from build123d import *

# Parameters (mm, degrees)
CROQUIS1_W              = 100
CROQUIS1_H              = 49
SALIENTE_EXTRUIR1_DEPTH = 40
CROQUIS2_W              = 70
CROQUIS2_H              = 29
CORTAR_EXTRUIR1_DEPTH   = 35
CORTAR_EXTRUIR2_DEPTH   = 14.9
CORTAR_EXTRUIR4_DEPTH   = 119.325821358
CROQUIS6_W              = 20.5
CROQUIS6_H              = 16.2
CORTAR_EXTRUIR6_DEPTH   = 119.325821358
CROQUIS7_W              = 58
CROQUIS7_H              = 18
SALIENTE_EXTRUIR2_DEPTH = 16
CROQUIS8_W              = 54
CROQUIS8_H              = 14
CORTAR_EXTRUIR7_DEPTH   = 16
ENVOLVER2_START         = -2.5
ENVOLVER2_DEPTH         = 2.5
CROQUIS11_W             = 75
CROQUIS11_H             = 10
SALIENTE_EXTRUIR3_DEPTH = 44
CROQUIS12_W             = 67
CROQUIS12_H             = 45
CORTAR_EXTRUIR8_DEPTH   = 5
CROQUIS13_W             = 71
CROQUIS13_H             = 1.5
CORTAR_EXTRUIR9_DEPTH   = 54
CROQUIS14_W             = 20
CROQUIS14_H             = 12
CORTAR_EXTRUIR10_DEPTH  = 5
CORTAR_EXTRUIR11_REACH  = 144.299
CROQUIS5_W              = 20.5
CROQUIS5_H              = 16.2
CROQUIS15_W             = 75
CROQUIS15_H             = 10
SALIENTE_EXTRUIR4_DEPTH = 1
CROQUIS16_W             = 75
CROQUIS16_H             = 14.9
CROQUIS16_W_2           = 15
CROQUIS16_H_2           = 25
CORTAR_EXTRUIR12_DEPTH  = 2.4
SALIENTE_EXTRUIR5_DEPTH = 2


# Read off the part's stored shape, not the designer's step: Envolver2
with BuildPart() as part:
    # Croquis1 → Saliente-Extruir1 (new body)
    with BuildSketch(Plane(origin=(0, 0, 0), x_dir=(1, 0, 0), z_dir=(0, 1, 0))):
        with Locations((50, 24.5)):
            Rectangle(CROQUIS1_W, CROQUIS1_H)
    extrude(amount=SALIENTE_EXTRUIR1_DEPTH)

    # Croquis2 → Cortar-Extruir1 (cut)
    with BuildSketch(Plane(origin=(0, 40, 0), x_dir=(1, 0, 0), z_dir=(0, 1, 0))):
        with Locations((50, 29.5)):
            Rectangle(CROQUIS2_W, CROQUIS2_H)
    extrude(amount=-CORTAR_EXTRUIR1_DEPTH, mode=Mode.SUBTRACT)

    # Croquis3 → Cortar-Extruir2 (cut)
    with BuildSketch(Plane.XY):
        Polygon((12.5, 5), (12.5, 25), (87.5, 25), (87.5, 5), (100, 5), (100, 40), (0, 40), (0, 5), align=None)
    extrude(amount=-CORTAR_EXTRUIR2_DEPTH, mode=Mode.SUBTRACT)

    # Croquis4 → Cortar-Extruir4 (cut, through all)
    with BuildSketch(Plane.ZY):
        Polygon((-44, 25), (-19, 25), (-19, 5), (-14.9, 5), (-14.9, 40), (-44, 40), align=None)
    extrude(amount=-CORTAR_EXTRUIR4_DEPTH, mode=Mode.SUBTRACT)

    # Croquis6 → Cortar-Extruir6 (cut, through all)
    with BuildSketch(Plane(origin=(100, 0, 0), x_dir=(0, 0, -1), z_dir=(1, 0, 0))):
        with Locations((31.75, 14.5)):
            Rectangle(CROQUIS6_W, CROQUIS6_H)
    extrude(amount=-CORTAR_EXTRUIR6_DEPTH, mode=Mode.SUBTRACT)

    # Croquis7 → Saliente-Extruir2 (add)
    with BuildSketch(Plane(origin=(0, 5, 0), x_dir=(1, 0, 0), z_dir=(0, 1, 0))):
        with Locations((50, 35)):
            Rectangle(CROQUIS7_W, CROQUIS7_H)
    extrude(amount=SALIENTE_EXTRUIR2_DEPTH)

    # Croquis8 → Cortar-Extruir7 (cut)
    with BuildSketch(Plane(origin=(0, 21, 0), x_dir=(1, 0, 0), z_dir=(0, 1, 0))):
        with Locations((50, 35)):
            Rectangle(CROQUIS8_W, CROQUIS8_H)
    extrude(amount=-CORTAR_EXTRUIR7_DEPTH, mode=Mode.SUBTRACT)

    # Envolver2 outline → Envolver2 (cut)
    # profile 1 of 3: a face of its own
    with BuildSketch(Plane(origin=(0, 5, 0), x_dir=(1, 0, 0), z_dir=(0, 1, 0)).offset(ENVOLVER2_START)):
        with BuildLine():
            add(Edge.make_bspline(
                [(44.845927513, 22.682039813), (44.880502524, 22.681581101), (44.94779002, 22.680688388), (45.045978034, 22.678103561), (45.138406194, 22.671034857), (45.225422346, 22.663758255), (45.306894242, 22.652117669), (45.382891805, 22.638865253), (45.453428219, 22.622573117), (45.519399834, 22.604194379), (45.582065701, 22.58175166), (45.642294727, 22.553081251), (45.700763218, 22.518735345), (45.757273689, 22.477750733), (45.813128977, 22.432374893), (45.865885411, 22.37921084), (45.918377238, 22.321807714), (45.967578278, 22.25830401), (46.01447324, 22.191680732), (46.054376208, 22.120908747), (46.088223994, 22.047966819), (46.117214563, 21.973058038), (46.136979973, 21.894799291), (46.154181469, 21.814812457), (46.162464556, 21.732060085), (46.163897144, 21.676148523), (46.164618555, 21.647993057)],
                knots=[0, 0, 0, 0, 0.054369818, 0.105810783, 0.1543913, 0.200099433, 0.243069893, 0.283740822, 0.321360744, 0.356845277, 0.391373506, 0.42587086, 0.461574928, 0.497826917, 0.535543491, 0.574581255, 0.615459073, 0.657779879, 0.700797841, 0.743450957, 0.785305491, 0.827181235, 0.869502041, 0.912065543, 0.955718718, 1, 1, 1, 1], degree=3))
            Line((44.845927513, 22.682039813), (43.424314244, 22.682039813))
            Line((43.424314244, 22.682039813), (42.805172718, 18.976839617))
            Line((42.805172718, 18.976839617), (43.469342719, 18.976839617))
            Line((43.469342719, 18.976839617), (43.718607489, 20.469211918))
            Line((43.718607489, 20.469211918), (44.603095383, 20.469211918))
            Line((44.603095383, 20.469211918), (45.04292709, 18.976839617))
            Line((45.04292709, 18.976839617), (45.752929645, 18.976839617))
            Line((45.752929645, 18.976839617), (45.28977962, 20.548011749))
            add(Edge.make_bspline(
                [(46.164618555, 21.647993057), (46.164091676, 21.617670303), (46.163039403, 21.5571103), (46.151744736, 21.467468845), (46.13622668, 21.379126232), (46.112503265, 21.292592771), (46.082048693, 21.207680933), (46.044780457, 21.124441143), (46.001130757, 21.043108672), (45.951712013, 20.9635574), (45.895224481, 20.887990565), (45.830214645, 20.819272615), (45.758276279, 20.757071565), (45.678885267, 20.701205138), (45.592072867, 20.652370985), (45.497799172, 20.610367641), (45.396617343, 20.574987864), (45.325850603, 20.557119534), (45.28977962, 20.548011749)],
                knots=[0, 0, 0, 0, 0.059520551, 0.118873267, 0.177208837, 0.235565778, 0.294841411, 0.354222133, 0.414510544, 0.476000381, 0.538010758, 0.599455515, 0.661405537, 0.724496825, 0.78978963, 0.856706752, 0.926961053, 1, 1, 1, 1], degree=3))
        make_face()
        with BuildLine():
            add(Edge.make_bspline(
                [(44.743809366, 21.03528417), (44.778129381, 21.03600119), (44.843652036, 21.0373701), (44.937526666, 21.044910102), (45.022020151, 21.059216882), (45.097465695, 21.079213334), (45.164300411, 21.104537257), (45.221481868, 21.136836672), (45.270624581, 21.17399479), (45.32077283, 21.232312946), (45.36864261, 21.310567266), (45.413007527, 21.407196099), (45.438530205, 21.507321555), (45.442292151, 21.574957755), (45.444162962, 21.608593141)],
                knots=[0, 0, 0, 0, 0.099664188, 0.190275618, 0.273183536, 0.348129931, 0.416633313, 0.480054439, 0.538277477, 0.594505454, 0.702244126, 0.80362549, 0.902343236, 1, 1, 1, 1], degree=3))
            Line((44.743809366, 21.03528417), (43.812684837, 21.03528417))
            Line((43.812684837, 21.03528417), (43.993602816, 22.115967561))
            Line((43.993602816, 22.115967561), (44.735768567, 22.115967561))
            add(Edge.make_bspline(
                [(45.444162962, 21.608593141), (45.443321191, 21.636863214), (45.441681994, 21.691914124), (45.421908744, 21.770970842), (45.392768442, 21.844328967), (45.35019923, 21.909220717), (45.300609579, 21.965653441), (45.246923641, 22.013950522), (45.187891151, 22.050903022), (45.122329195, 22.077622199), (45.046506806, 22.09459194), (44.957252302, 22.107151834), (44.85196106, 22.115045121), (44.776255138, 22.115646142), (44.735768567, 22.115967561)],
                knots=[0, 0, 0, 0, 0.084973229, 0.165470167, 0.24404472, 0.32176826, 0.397881214, 0.469968558, 0.538528016, 0.606605512, 0.682202732, 0.771959831, 0.878046995, 1, 1, 1, 1], degree=3))
        make_face(mode=Mode.SUBTRACT)
    # profile 2 of 3: a face of its own
    with BuildSketch(Plane(origin=(0, 5, 0), x_dir=(1, 0, 0), z_dir=(0, 1, 0)).offset(ENVOLVER2_START)):
        Polygon((46.976739258, 22.682039813), (46.357597732, 18.976839617), (48.79395984, 18.976839617), (48.892057588, 19.542911869), (47.113432841, 19.542911869), (47.285505941, 20.572134146), (48.696666171, 20.572134146), (48.78913536, 21.138206398), (47.379583289, 21.138206398), (47.54281151, 22.115967561), (49.257109864, 22.115967561), (49.355207612, 22.682039813), align=None)
    # profile 3 of 3: a face of its own
    with BuildSketch(Plane(origin=(0, 5, 0), x_dir=(1, 0, 0), z_dir=(0, 1, 0)).offset(ENVOLVER2_START)):
        Polygon((50.984273497, 22.682039813), (49.96148386, 22.682039813), (49.342342334, 18.976839617), (49.858561632, 18.976839617), (50.417397165, 22.321007936), (50.952914381, 18.976839617), (51.313946257, 18.976839617), (52.891551028, 22.350758892), (52.327086936, 18.976839617), (52.991256936, 18.976839617), (53.611202541, 22.682039813), (52.559466028, 22.682039813), (51.387921608, 20.172506434), align=None)
    extrude(amount=ENVOLVER2_DEPTH, mode=Mode.SUBTRACT)

    # Croquis11 → Saliente-Extruir3 (add)
    with BuildSketch(Plane(origin=(0, 0, -49), x_dir=(-1, 0, 0), z_dir=(0, 0, -1))):
        with Locations((-50, 35)):
            Rectangle(CROQUIS11_W, CROQUIS11_H)
    extrude(amount=SALIENTE_EXTRUIR3_DEPTH)

    # Croquis12 → Cortar-Extruir8 (cut)
    with BuildSketch(Plane(origin=(0, 40, 0), x_dir=(1, 0, 0), z_dir=(0, 1, 0))):
        with Locations((50, 66.5)):
            Rectangle(CROQUIS12_W, CROQUIS12_H)
    extrude(amount=-CORTAR_EXTRUIR8_DEPTH, mode=Mode.SUBTRACT)

    # Croquis13 → Cortar-Extruir9 (cut)
    with BuildSketch(Plane.XY.offset(-44)):
        with Locations((50, 37.5)):
            Rectangle(CROQUIS13_W, CROQUIS13_H)
    extrude(amount=-CORTAR_EXTRUIR9_DEPTH, mode=Mode.SUBTRACT)

    # Croquis14 → Cortar-Extruir10 (cut)
    with BuildSketch(Plane(origin=(0, 35, 0), x_dir=(1, 0, 0), z_dir=(0, 1, 0))):
        with Locations((50.5, 80)):
            Rectangle(CROQUIS14_W, CROQUIS14_H)
    extrude(amount=-CORTAR_EXTRUIR10_DEPTH, mode=Mode.SUBTRACT)

    # Croquis5 → Cortar-Extruir11 (cut, up to next)
    with BuildSketch(Plane.XY, mode=Mode.PRIVATE) as cortar_extruir11_sk1:
        with Locations((26.25, 14.5)):
            Rectangle(CROQUIS5_W, CROQUIS5_H)
    cortar_extruir11_tool1 = extrude(cortar_extruir11_sk1.sketch, amount=-CORTAR_EXTRUIR11_REACH, mode=Mode.PRIVATE) & part.part
    # Croquis5 → Cortar-Extruir11 (cut, up to next)
    with BuildSketch(Plane.XY, mode=Mode.PRIVATE) as cortar_extruir11_sk2:
        with Locations((50, 14.5)):
            Rectangle(CROQUIS5_W, CROQUIS5_H)
    cortar_extruir11_tool2 = extrude(cortar_extruir11_sk2.sketch, amount=-CORTAR_EXTRUIR11_REACH, mode=Mode.PRIVATE) & part.part
    # Croquis5 → Cortar-Extruir11 (cut, up to next)
    with BuildSketch(Plane.XY, mode=Mode.PRIVATE) as cortar_extruir11_sk3:
        with Locations((73.75, 14.5)):
            Rectangle(CROQUIS5_W, CROQUIS5_H)
    cortar_extruir11_tool3 = extrude(cortar_extruir11_sk3.sketch, amount=-CORTAR_EXTRUIR11_REACH, mode=Mode.PRIVATE) & part.part
    add(cortar_extruir11_tool1.solids().sort_by_distance((26.25, 14.5, 0))[0], mode=Mode.SUBTRACT)
    add(cortar_extruir11_tool2.solids().sort_by_distance((50, 14.5, 0))[0], mode=Mode.SUBTRACT)
    add(cortar_extruir11_tool3.solids().sort_by_distance((73.75, 14.5, 0))[0], mode=Mode.SUBTRACT)

    # Croquis15 → Saliente-Extruir4 (add)
    with BuildSketch(Plane(origin=(0, 0, -93), x_dir=(-1, 0, 0), z_dir=(0, 0, -1))):
        with Locations((-50, 35)):
            Rectangle(CROQUIS15_W, CROQUIS15_H)
    extrude(amount=SALIENTE_EXTRUIR4_DEPTH)

    # Croquis16 → Cortar-Extruir12 (cut)
    with BuildSketch(Plane(origin=(0, 25, 0), x_dir=(1, 0, 0), z_dir=(0, 1, 0))):
        with Locations((50, 7.45)):
            Rectangle(CROQUIS16_W, CROQUIS16_H)
        with Locations((7.5, 31.5)):
            Rectangle(CROQUIS16_W_2, CROQUIS16_H_2)
        with Locations((92.5, 31.5)):
            Rectangle(CROQUIS16_W_2, CROQUIS16_H_2)
    extrude(amount=-CORTAR_EXTRUIR12_DEPTH, mode=Mode.SUBTRACT)

    # Croquis17 → Saliente-Extruir5 (add)
    with BuildSketch(Plane.XY.offset(-44)):
        Polygon((0, 40), (16.5, 40), (16.5, 38.25), (14.5, 38.25), (14.5, 36.75), (16.5, 36.75), (16.5, 35), (83.5, 35), (83.5, 36.75), (85.5, 36.75), (85.5, 38.25), (83.5, 38.25), (83.5, 40), (100, 40), (100, 22.6), (85, 22.6), (85, 5), (79, 5), (79, 21), (21, 21), (21, 5), (15, 5), (15, 22.6), (0, 22.6), align=None)
    extrude(amount=SALIENTE_EXTRUIR5_DEPTH)


solid = part.part
Verification items for the finished model (mm, model axes). A direction names the side the tool comes from. Give positions to 0.01 mm unless a question says otherwise; leave off trailing zeros. Loops run counter-clockwise (first coordinate to the right, second up) from the corner with the lowest first, then second, coordinate; pieces in that order, holes last.
1) Sectioned sample at B-B, the plane x = 70.5. Enter the section's corners in (y, z).
2) Sectioned sample at D-D, the plane z = -62. Enter the section's corners in (x, y).
3) Thickness scan on line 1 along Z through (x, y) = (14.5, 19.5); line 2 along Z through (x, y) = (48.5, 3.5); line 3 along X through (y, z) = (18, -39). Record the ranges inside material, lowest first.
4) Depth check by flat-ended pin: pin 1 Ø3 at (x, z) = (14, -7) entering from +Y; pin 2 Ø4.5 at (y, z) = (11.5, -11) entering from -X; pin 3 Ø7.5 at (x, z) = (48.5, -8) entering from +Y. Enter the tip coordinate at first touch or a pass-through.
5) Set-up check for faces 3 (the flat face through (93, 6.4, -32)), 4 (the flat face through (53, 6, -14.9)), 5 (the flat face through (92, 22.6, -20)), 6 (the flat face through (51, 30, -71)): record each of +Z, -Z, +X, -X, +Y, -Y from which the full face is reachable in a straight line by a thin tool's end or side.
6) Sectioned sample at A-A, the plane z = -38.5. Enter the section's corners in (x, y).
7) Sectioned sample at C-C, the plane y = 17. Count the separate pieces of the cut face and the enclosed holes in it, then the cut area to 3 significant figures.
8) Draft check along Z on faces 1 (the flat face through (46.672, 3.732, -20.855)), 2 (the flat face through (86, 22.6, -8)). Enter one of: pulls with the +Z half, pulls with the -Z half, needs draft (parallel to the pull), parting line crosses it, or undercut.
Answers:
1. outline: (0, -49) - (30, -49) - (30, -94) - (40, -94) - (40, -89) - (38.25, -89) - (38.25, -93) - (36.75, -93) - (36.75, -89) - (35, -89) - (35, -42) - (5, -42) - (5, -28) - (21, -28) - (21, -26) - (5, -26) - (5, -14.9) - (6.4, -14.9) - (6.4, 0) - (0, 0) - close
2. outline: (12.5, 30) - (87.5, 30) - (87.5, 40) - (83.5, 40) - (83.5, 38.25) - (85.5, 38.25) - (85.5, 36.75) - (83.5, 36.75) - (83.5, 35) - (16.5, 35) - (16.5, 36.75) - (14.5, 36.75) - (14.5, 38.25) - (16.5, 38.25) - (16.5, 40) - (12.5, 40) - close
3. line 1: z = -49 to -42, -21.5 to -19, -14.9 to 0
3. line 2: z = -49 to -22.68, -22.12 to -21.14, -20.57 to -19.54, -18.98 to 0
3. line 3: x = 21 to 23, 77 to 79
4. pin 1: stops at y = 22.6
4. pin 2: stops at x = 12.5
4. pin 3: stops at y = 6.4
5. face 3: +X, +Y
5. face 4: +X, -X, +Y
5. face 5: +Z, +X, -X, +Y
5. face 6: -Z, +X, -X, -Y
6. outline: (0, 0) - (100, 0) - (100, 6.4) - (85, 6.4) - (85, 5) - (79, 5) - (79, 21) - (77, 21) - (77, 5) - (23, 5) - (23, 21) - (21, 21) - (21, 5) - (15, 5) - (15, 6.4) - (0, 6.4) - close
7. separate pieces: 7
7. enclosed holes: 1
7. area: 1,150 mm2
8. face 1: undercut
8. face 2: needs draft
